from build123d import *

# Parameters (mm, degrees)
SKETCH1_W                = 120
SKETCH1_H                = 34
BOSS_EXTRUDE1_DEPTH      = 5
CUT_EXTRUDE1_DEPTH       = 2.5
M3_CLEARANCE_HOLE1_D     = 3.4
M3_CLEARANCE_HOLE1_DEPTH = 15
M3_CLEARANCE_HOLE1_TIP   = 1.021463052
M3_CLEARANCE_HOLE3_D     = 3.4
M3_CLEARANCE_HOLE3_DEPTH = 15
M3_CLEARANCE_HOLE3_TIP   = 1.021463052


with BuildPart() as part:
    # Sketch1 → Boss-Extrude1 (new body)
    with BuildSketch(Plane(origin=(0, 0, 0), x_dir=(0, 0, -1), z_dir=(1, 0, 0))):
        with Locations((-60, 17)):
            Rectangle(SKETCH1_W, SKETCH1_H)
    extrude(amount=BOSS_EXTRUDE1_DEPTH)

    # Sketch2 → Cut-Extrude1 (cut)
    with BuildSketch(Plane(origin=(5, 0, 0), x_dir=(0, 0, -1), z_dir=(1, 0, 0))):
        with BuildLine():
            ThreePointArc((-45.85, 17), (-49.994439046, 27.005560954), (-60, 31.15))
            Line((-60, 31.15), (-60, 2.85))
            ThreePointArc((-60, 2.85), (-49.994439046, 6.994439046), (-45.85, 17))
        make_face()
        with BuildLine():
            Line((-60, 2.85), (-60, 31.15))
            ThreePointArc((-60, 31.15), (-74.15, 17), (-60, 2.85))
        make_face()
    extrude(amount=-CUT_EXTRUDE1_DEPTH, mode=Mode.SUBTRACT)

    # M3 Clearance Hole1
    with Locations(Plane(origin=(2.5, 0, 0), x_dir=(0, 0, -1), z_dir=(1, 0, 0))):
        with Locations((-60, 27.8), (-49.2, 17), (-60, 6.2), (-70.8, 17)):
            Hole(M3_CLEARANCE_HOLE1_D / 2, depth=M3_CLEARANCE_HOLE1_DEPTH)
            with Locations((0, 0, -(M3_CLEARANCE_HOLE1_DEPTH + M3_CLEARANCE_HOLE1_TIP / 2))):  # 118° drill point
                Cone(0, M3_CLEARANCE_HOLE1_D / 2, M3_CLEARANCE_HOLE1_TIP, mode=Mode.SUBTRACT)

    # M3 Clearance Hole3
    with Locations(Plane.ZY):
        with Locations((24, 11), (13, 4), (96, 11), (107, 4)):
            Hole(M3_CLEARANCE_HOLE3_D / 2, depth=M3_CLEARANCE_HOLE3_DEPTH)
            with Locations((0, 0, -(M3_CLEARANCE_HOLE3_DEPTH + M3_CLEARANCE_HOLE3_TIP / 2))):  # 118° drill point
                Cone(0, M3_CLEARANCE_HOLE3_D / 2, M3_CLEARANCE_HOLE3_TIP, mode=Mode.SUBTRACT)


solid = part.part
Geometry check sheet. Reference: the model listing, model coordinates, mm. A direction names the side the tool comes from. Coordinates: 2 decimals unless noted, no trailing zeros. Order: outer loops, then holes, each group sorted by start corner. A loop starts at its lowest first (then second) coordinate and runs counter-clockwise, first axis right, second up. Notation, with made-up numbers: (34.5, 25) -> (53.5, 25) arc R29 cw to (53.5, 63) -> close; hole circle Ø10 at (19, 51.5). An arc over 180 degrees is marked (long way). Use a Markdown table: item, result. Add a question column.
1. Cross-section at C-C (y = 27.8). Enter the section's corners in (x, z), and give its area (3 significant figures).
2. Cross-section at B-B (x = 1.15). Give the number of separate pieces and of enclosed holes in the cut face, and give its area (3 significant figures).
3. Go/stop test with a flat-tipped pin: pin 1 Ø5.5 at (y, z) = (6.2, 60) entering from +X. Record where the tip stops, or that it passes through.
4. Material ranges on L1, parallel to Y at x = 0.9, z = 60; L2, parallel to Z at x = 1.95, y = 6; L3, parallel to Y at x = 1.8, z = 49.2, recorded low to high.
5. Cross-section at A-A (z = 24). Enter the section's corners in (x, y), and give its area (3 significant figures).
6. Set-up check for faces 1 (the face through (2.5, 17, 60)), 2 (the face through (2.54, 11.07, 97.7)): record each of +Z, -Z, +X, -X, +Y, -Y from which the full face is reachable in a straight line by a thin tool's end or side.
7. Mould release check, pull along Y, two halves, no side actions. Record for faces 3 (the face through (5, 21, 74)), 4 (the face through (1.23, 17.07, 69.1)), 5 (the face through (2, 34, 61)): pulls with the +Y half, pulls with the -Y half, needs draft (parallel to the pull), parting line crosses it, or undercut.
8. Cross-section at D-D (z = 52). Enter the section's corners in (x, y).
Filled sheet:
| question | item | result |
|---|---|---|
| 1 | outline | (0, 0) -> (5, 0) -> (5, 50.86) -> (2.5, 50.86) -> (2.5, 58.3) -> (0, 58.3) -> close; (0, 61.7) -> (2.5, 61.7) -> (2.5, 69.14) -> (5, 69.14) -> (5, 120) -> (0, 120) -> close |
| 1 | area | 546 mm2 |
| 2 | separate pieces | 1 |
| 2 | enclosed holes | 8 |
| 2 | area | 4,010 mm2 |
| 3 | pin 1 | x = 2.5 |
| 4 | L1 | 0 to 4.5, 7.9 to 26.1, 29.5 to 34 |
| 4 | L2 | 0 to 58.31, 61.69 to 120 |
| 4 | L3 | 0 to 15.3, 18.7 to 34 |
| 5 | outline | (0, 0) -> (5, 0) -> (5, 9.3) -> (0, 9.3) -> close; (0, 12.7) -> (5, 12.7) -> (5, 34) -> (0, 34) -> close |
| 5 | area | 153 mm2 |
| 6 | face 1 | +X |
| 6 | face 2 | +X, -X |
| 7 | face 3 | needs draft |
| 7 | face 4 | undercut |
| 7 | face 5 | pulls with the +Y half |
| 8 | outline | (0, 0) -> (5, 0) -> (5, 5.33) -> (2.5, 5.33) -> (2.5, 28.67) -> (5, 28.67) -> (5, 34) -> (0, 34) -> close |
